The drawing under review shows one solid part. Ordinate dimensions are in mm from its lowest x, y, z. A direction names the side the tool comes from. Coordinates: 2 decimals unless noted, no trailing zeros. Write each loop counter-clockwise with the first axis right and the second up, starting at its lowest first coordinate (ties: lowest second). Pieces come first, ordered by that corner, then holes.
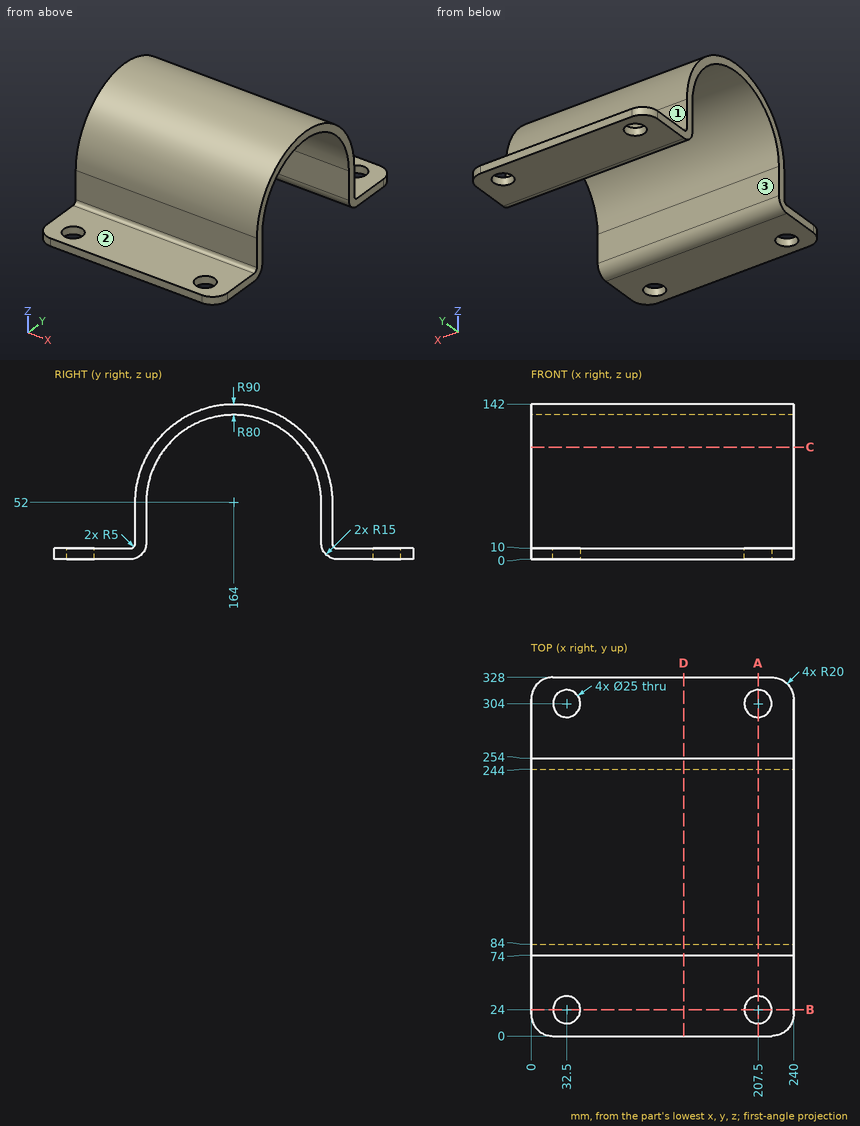
Q1. For probe 1 along Y at (x, z) = (115, 40); probe 2 along Y at (x, z) = (207, 4); probe 3 along Y at (x, z) = (207.5, 6.5), list the stretches that pass through material, from the lowest coordinate up.
Ans:
probe 1: y = 74 to 84, 244 to 254
probe 2: y = 0 to 11.51, 36.49 to 79.2, 248.8 to 291.51, 316.49 to 328
probe 3: y = 0 to 11.5, 36.5 to 81.36, 246.64 to 291.5, 316.5 to 328
Q2. Add section D-D (x = 139.5). State the section outline as (y, z) points.
Ans:
outline: (0, 0) - (69, 0) arc R15 ccw to (84, 15) - (84, 52) arc R80 cw to (244, 52) - (244, 15) arc R15 ccw to (259, 0) - (328, 0) - (328, 10) - (259, 10) arc R5 cw to (254, 15) - (254, 52) arc R90 ccw to (74, 52) - (74, 15) arc R5 cw to (69, 10) - (0, 10) - close
Q3. Add section B-B (y = 24). State the section outline as (x, z) points.
Ans:
outline: (0, 0) - (20, 0) - (20, 10) - (0, 10) - close; (45, 0) - (195, 0) - (195, 10) - (45, 10) - close; (220, 0) - (240, 0) - (240, 10) - (220, 10) - close
Q4. Add section C-C (z = 102.5). State the section outline as (x, y) points, then the cut area to 3 significant figures.
Ans:
outline: (0, 89.5) - (240, 89.5) - (240, 101.95) - (0, 101.95) - close; (0, 226.05) - (240, 226.05) - (240, 238.5) - (0, 238.5) - close
area: 5,980 mm2
Q5. Add section A-A (x = 207.5). State the section outline as (y, z) points.
Ans:
outline: (0, 0) - (11.5, 0) - (11.5, 10) - (0, 10) - close; (36.5, 0) - (69, 0) arc R15 ccw to (84, 15) - (84, 52) arc R80 cw to (244, 52) - (244, 15) arc R15 ccw to (259, 0) - (291.5, 0) - (291.5, 10) - (259, 10) arc R5 cw to (254, 15) - (254, 52) arc R90 ccw to (74, 52) - (74, 15) arc R5 cw to (69, 10) - (36.5, 10) - close; (316.5, 0) - (328, 0) - (328, 10) - (316.5, 10) - close
Q6. Clearance check with flat-ended pins moving along their axes: pin 1 Ø4 at (x, z) = (112.5, 31.5) entering from -Y; pin 2 Ø20.5 at (x, y) = (83, 285.5) entering from +Z; pin 3 Ø3 at (x, z) = (204, 59) entering from +Y. State where each tip first meets the part, or that it passes through.
Ans:
pin 1: stops at y = 74
pin 2: stops at z = 10
pin 3: stops at y = 253.83
Q7. Tool access review of the marked faces 1, 2 and 3: name each direction out of +Z, -Z, +X, -X, +Y, -Y from which nothing blocks a thin tool from reaching the whole face with its end or side.
Ans:
face 1: +Z, +X, -X, +Y
face 2: +Z, +X, -X, -Y
face 3: -Z, +X, -X
